from build123d import *

# Parameters (mm, degrees)
F0_R     = 10
F1_DEPTH = 3
F2_R     = 6.25
F3_DEPTH = 21
F4_R     = 4.15
F5_DEPTH = 25
F6_SIZE2 = 2
F6_SIZE  = 1


with BuildPart() as f1:
    # F0 (on Top) → F1 (new body)
    with BuildSketch(Plane.XY):
        Circle(F0_R)
    extrude(amount=F1_DEPTH)

    # F2 (on face) → F3 (join)
    with BuildSketch(Plane.XY.offset(3)):
        Circle(F2_R)
    extrude(amount=F3_DEPTH)

    # F4 (on face) → F5 (cut)
    with BuildSketch(Plane.XY.offset(24)):
        Circle(F4_R)
    extrude(amount=-F5_DEPTH, mode=Mode.SUBTRACT)

    # F6
    f6_edges = [f1.edges().sort_by_distance(p)[0] for p in [
        (-6.25, 0, 24),
    ]]
    f6_side = f1.faces().sort_by_distance((-6.073223, 0, 24))[0]
    chamfer(f6_edges, length=F6_SIZE, length2=F6_SIZE2, reference=f6_side)


solid = f1.part
The listing builds one solid part. Answer for the finished solid, in the listing's coordinates (mm). Give positions to 0.01 mm unless a question says otherwise; leave off trailing zeros. Loops run counter-clockwise (first coordinate to the right, second up) from the corner with the lowest first, then second, coordinate; pieces in that order, holes last. Notation, with made-up numbers: (-25, 42.25) - (24, 42.25) arc R17 cw to (24, 57.25) - close; hole circle Ø2 at (30.5, 12.5). An arc over 180 degrees is marked (long way). Use one line per item in the form item = value.
1. The mould has two halves that part along X. Classify faces 1 (the face through (-0.9, -4.05, 12.17)), 2 (the face through (4, 5, 3)), 3 (the face through (5.96, 1.88, 12.37)): pulls with the +X half, pulls with the -X half, needs draft (parallel to the pull), parting line crosses it, or undercut.
Calculated:
face_1 = undercut
face_2 = needs draft
face_3 = parting line crosses it
2. Section D-D on y = -8 is taken. Give the vertices of the cut face in (x, z), then the cut area to 3 significant figures.
Calculated:
outline = (-6, 0) - (6, 0) - (6, 3) - (-6, 3) - close
area = 36.0 mm^2
3. Given pin 1 Ø2 at (x, z) = (3.5, 7.5) entering from -Y; pin 2 Ø5 at (x, y) = (7.5, 2.5) entering from -Z; pin 3 Ø12 at (x, z) = (2, 17.5) entering from -Y; pin 4 Ø6 at (x, z) = (8, 11.5) entering from -Y, each flat-ended and moving along its own axis, determine where each tip first touches the part or whether it passes through.
Calculated:
pin_1 = -5.73
pin_2 = 0
pin_3 = -6.25
pin_4 = -3.75
4. Section A-A on y = 0 is taken. Give the vertices of the cut face in (x, z), then the cut area to 3 significant figures.
Calculated:
outline = (-10, 0) - (-4.15, 0) - (-4.15, 24) - (-5.25, 24) - (-6.25, 22) - (-6.25, 3) - (-10, 3) - close; (4.15, 0) - (10, 0) - (10, 3) - (6.25, 3) - (6.25, 22) - (5.25, 24) - (4.15, 24) - close
area = 121 mm^2
5. Section C-C on z = 14.75 is taken. Give the vertices of the cut face in (x, y).
Calculated:
outline = circle Ø12.5 at (0, 0); hole circle Ø8.3 at (0, 0)
6. Find the intervals of material crossed by line 1 along Y through (x, z) = (0, 16.25); line 2 along Z through (x, y) = (5, 8.25); line 3 along Y through (x, z) = (-3.5, 4), in increasing order. Write a range as [from, to].
Calculated:
line_1 = [-6.25, -4.15], [4.15, 6.25]
line_2 = [0, 3]
line_3 = [-5.18, -2.23], [2.23, 5.18]
